The model under review builds one solid part; all positions refer to its coordinate system, in mm. A direction names the side the tool comes from. Give positions to 0.01 mm unless a question says otherwise; leave off trailing zeros. Order: outer loops, then holes, each group sorted by start corner. A loop starts at its lowest first (then second) coordinate and runs counter-clockwise, first axis right, second up. Notation, with made-up numbers: (55, 38) - (80, 38) arc R14 cw to (80, 53) - close; hole circle Ø4 at (3.25, 29). An arc over 180 degrees is marked (long way). Write item = value, one per line. Start each with the question number.
1. We need section A-A, the plane z = -230. Give the boundary of the cut face in (x, y).
2. We need section D-D, the plane z = -125. Give the boundary of the cut face in (x, y).
3. Mouldability with a two-part tool opening along Z and no side actions: class faces 5 (the flat face through (225, -3, -250)), 6 (the flat face through (197, -3, -78)), 7 (the flat face through (151, -6, -127)) as pulls with the +Z half, pulls with the -Z half, needs draft (parallel to the pull), parting line crosses it, or undercut.
4. For P1, Ø1.5, axis at y = -1.5, z = -104.5, coming from the -X side; P2, Ø1.5, axis at y = -1.5, z = -100.5, coming from the -X side; P3, Ø1.8, axis at y = -3.5, z = -123, coming from the -X side, all flat-tipped, find the tip position at first contact; note any pin that passes through.
5. We need section B-B, the plane x = 20. Give the boundary of the cut face in (y, z), and give its area (3 significant figures).
6. Wall thickness on probe 1 along Z at (x, y) = (230, -1.5); probe 2 along X at (y, z) = (-4.4, -230); probe 3 along X at (y, z) = (-1.8, -125): over which ranges is each line inside the solid? List them lowest first.
7. We need section C-C, the plane x = 188. Give the boundary of the cut face in (y, z), and give its area (3 significant figures).
8. Machinability: for faces 1 (the flat face through (50, -3, -237)), 2 (the flat face through (172, -3, -53)), 3 (the flat face through (52, -3, -173)), 4 (the flat face through (237, -3, -50)), which of the approach directions +Z, -Z, +X, -X, +Y, -Y give a long, thin tool a straight path to every point of the face, cutting with its end or side? Answer none if there is none.
from build123d import *

# Parameters (mm, degrees)
SKETCH1_W   = 250
SKETCH1_H   = 250
TABLE_DEPTH = 6
SKETCH2_R   = 3.25
CUT_DEPTH   = 6
FILLET1_R   = 1
SKETCH3_R   = 20
LITE_DEPTH  = 354.604298616


with BuildPart() as part:
    # Sketch1 → table (new body)
    with BuildSketch(Plane(origin=(0, 0, 0), x_dir=(1, 0, 0), z_dir=(0, 1, 0))):
        with Locations((125, 125)):
            Rectangle(SKETCH1_W, SKETCH1_H)
    extrude(amount=-TABLE_DEPTH)

    # Sketch2 → cut (cut)
    with BuildSketch(Plane(origin=(0, 0, 0), x_dir=(1, 0, 0), z_dir=(0, 1, 0))):
        with Locations(Location((20, 230, 0), (0, 0, 270))):
            Circle(SKETCH2_R)
        with Locations(Location((230, 230, 0), (0, 0, 270))):
            Circle(SKETCH2_R)
        with Locations(Location((230, 20, 0), (0, 0, 270))):
            Circle(SKETCH2_R)
        with Locations(Location((20, 20, 0), (0, 0, 270))):
            Circle(SKETCH2_R)
        Polygon((0, 200), (25, 200), (80, 145), (80, 105), (25, 50), (0, 50), align=None)
        Polygon((50, 250), (50, 225), (105, 170), (145, 170), (200, 225), (200, 250), align=None)
        Polygon((250, 200), (225, 200), (170, 145), (170, 105), (225, 50), (250, 50), align=None)
        Polygon((50, 0), (50, 25), (105, 80), (145, 80), (200, 25), (200, 0), align=None)
    extrude(amount=-CUT_DEPTH, mode=Mode.SUBTRACT)

    # Fillet1
    fillet1_edges = [part.edges().sort_by_distance(p)[0] for p in [
        (0, -3, -50),
        (0, -3, -200),
        (25, -3, -200),
        (80, -3, -145),
        (80, -3, -105),
        (25, -3, -50),
        (50, -3, -250),
        (200, -3, -250),
        (200, -3, -225),
        (145, -3, -170),
        (105, -3, -170),
        (50, -3, -225),
        (250, -3, -200),
        (250, -3, -50),
        (225, -3, -50),
        (170, -3, -105),
        (170, -3, -145),
        (225, -3, -200),
        (0, -3, -250),
        (250, -3, -250),
        (250, -3, 0),
        (0, -3, 0),
        (200, -3, 0),
        (50, -3, 0),
        (50, -3, -25),
        (105, -3, -80),
        (145, -3, -80),
        (200, -3, -25),
    ]]
    fillet(fillet1_edges, radius=FILLET1_R)

    # Sketch3 → lite (cut, through all)
    with BuildSketch(Plane(origin=(0, 0, 0), x_dir=(1, 0, 0), z_dir=(0, 1, 0))):
        with Locations(Location((125, 125, 0), (0, 0, 270))):
            Circle(SKETCH3_R)
    extrude(amount=-LITE_DEPTH, mode=Mode.SUBTRACT)


solid = part.part
Model answer:
q1.outline = (0, -6) - (16.75, -6) - (16.75, 0) - (0, 0) - close; (23.25, -6) - (50, -6) - (50, 0) - (23.25, 0) - close; (200, -6) - (226.75, -6) - (226.75, 0) - (200, 0) - close; (233.25, -6) - (250, -6) - (250, 0) - (233.25, 0) - close
q2.outline = (80, -6) - (105, -6) - (105, 0) - (80, 0) - close; (145, -6) - (170, -6) - (170, 0) - (145, 0) - close
q3.face_5 = pulls with the -Z half
q3.face_6 = undercut
q3.face_7 = needs draft
q4.P1 = 78.75
q4.P2 = 74.75
q4.P3 = 80
q5.outline = (-6, -250) - (0, -250) - (0, -233.25) - (-6, -233.25) - close; (-6, -226.75) - (0, -226.75) - (0, -200) - (-6, -200) - close; (-6, -50) - (0, -50) - (0, -23.25) - (-6, -23.25) - close; (-6, -16.75) - (0, -16.75) - (0, 0) - (-6, 0) - close
q5.area = 522 mm2
q6.probe_1 = -250 to -233.25, -226.75 to -200, -50 to -23.25, -16.75 to 0
q6.probe_2 = 0 to 16.75, 23.25 to 50, 200 to 226.75, 233.25 to 250
q6.probe_3 = 80 to 105, 145 to 170
q7.outline = (-6, -213) - (0, -213) - (0, -163) - (-6, -163) - close; (-6, -87) - (0, -87) - (0, -37) - (-6, -37) - close
q7.area = 600 mm2
q8.face_1 = -Z, +Y, -Y
q8.face_2 = +Z, +Y, -Y
q8.face_3 = -X, +Y, -Y
q8.face_4 = +X, +Y, -Y
